Check sheet for the modelled part. Datum: model origin and axes. Units: mm. Give positions to 0.01 mm unless a question says otherwise; leave off trailing zeros. Loops run counter-clockwise (first coordinate to the right, second up) from the corner with the lowest first, then second, coordinate; pieces in that order, holes last. Notation, with made-up numbers: (-12, 77.5) - (4, 77.5) arc R31 cw to (4, 105.5) - close; hole circle Ø5 at (42.25, 41.25). An arc over 180 degrees is marked (long way). Use CSV: the item, a comma, the result in double quotes.
from build123d import *

# Parameters (mm, degrees)
BOSS_EXTRUDE1_DEPTH      = 320.675
BOSS_EXTRUDE1_DEPTH_BACK = 320.675
SKETCH3_W                = 50.8
SKETCH3_H                = 25.4
SKETCH3_W_2              = 44.45
SKETCH3_H_2              = 19.05
CUT_EXTRUDE1_DEPTH       = 323.680609311
CUT_EXTRUDE1_DEPTH_BACK  = 323.680609311


with BuildPart() as part:
    # Sketch3 → Boss-Extrude1 (new, two sides: drawn at the far end of the back side and taken through both)
    with BuildSketch(Plane.XY.offset(-BOSS_EXTRUDE1_DEPTH_BACK)):
        Rectangle(SKETCH3_W, SKETCH3_H)
        Rectangle(SKETCH3_W_2, SKETCH3_H_2, mode=Mode.SUBTRACT)
    extrude(amount=BOSS_EXTRUDE1_DEPTH + BOSS_EXTRUDE1_DEPTH_BACK)

    # Sketch4 → Cut-Extrude1 (cut, two sides: drawn at the far end of the back side and taken through both)
    with BuildSketch(Plane(origin=(0, 12.7, 0), x_dir=(1, 0, 0), z_dir=(0, 1, 0)).offset(-CUT_EXTRUDE1_DEPTH_BACK)):
        Polygon((1322.117470931, -320.675), (25.4, -320.675), (-25.4, -320.675), (25.4, -305.627354456), (1268.718301677, 62.660305034), (3837.350959621, 420.474595165), (3890.750128875, 37.139290131), align=None)
    extrude(amount=CUT_EXTRUDE1_DEPTH + CUT_EXTRUDE1_DEPTH_BACK, mode=Mode.SUBTRACT)


solid = part.part
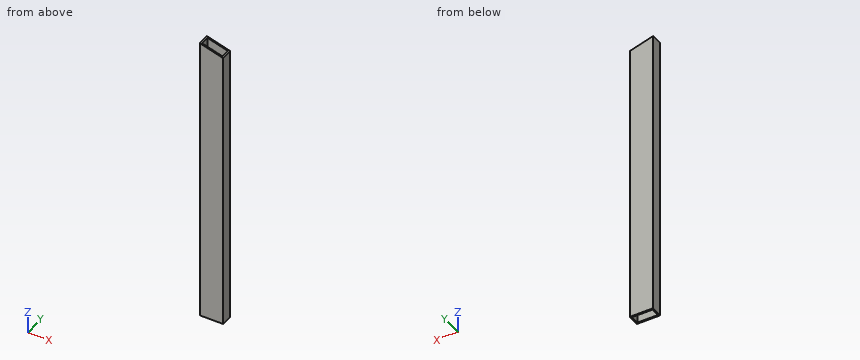
1. Sectioned sample at A-A, the plane z = 183. Record the boundary of the cut face in (x, y) (3 decimals), and give its area (3 significant figures).
Completed:
outline,"(-25.4, -12.7) - (25.4, -12.7) - (25.4, 12.7) - (-25.4, 12.7) - close; hole (-22.225, -9.525) - (22.225, -9.525) - (22.225, 9.525) - (-22.225, 9.525) - close"
area,"444 mm²"
2. Sectioned sample at B-B, the plane y = 0.5. Record the boundary of the cut face in (x, z) (3 decimals).
Completed:
outline,"(-25.4, -320.675) - (-22.225, -320.675) - (-22.225, 319.735) - (-25.4, 320.675) - close; (22.225, -320.675) - (25.4, -320.675) - (25.4, 305.627) - (22.225, 306.568) - close"
3. Go/stop test with flat-tipped pins: pin 1 Ø12 at (x, y) = (-0.5, -8) entering from -Z (3 decimals); pin 2 Ø5 at (x, y) = (0, 7.5) entering from +Z. Record where each tip stops, or that it passes through.
Completed:
pin 1,"stops at z = -320.675"
pin 2,"stops at z = 313.59"
4. Sectioned sample at C-C, the plane x = 11. Record the boundary of the cut face in (y, z) (3 decimals), and give its area (3 significant figures).
Completed:
outline,"(-12.7, -320.675) - (-9.525, -320.675) - (-9.525, 309.893) - (-12.7, 309.893) - close; (9.525, -320.675) - (12.7, -320.675) - (12.7, 309.893) - (9.525, 309.893) - close"
area,"4,000 mm²"
5. Scan lines: line 1 along Y through (x, z) = (-10, 65.5) (3 decimals); line 2 along X through (y, z) = (2.25, -71) (3 decimals); line 3 along Z through (x, y) = (-4, -11.25) (3 decimals). Record each from-to range of solid material in increasing order.
Completed:
line 1,"y = -12.7 to -9.525, 9.525 to 12.7"
line 2,"x = -25.4 to -22.225, 22.225 to 25.4"
line 3,"z = -320.675 to 314.336"
